Could you check a few things on this drawing? It's one solid part, dimensions in mm from its lowest x, y, z. Give positions to 0.01 mm unless a question says otherwise; leave off trailing zeros. Loops run counter-clockwise (first coordinate to the right, second up) from the corner with the lowest first, then second, coordinate; pieces in that order, holes last.
1. For P1, Ø6, axis at x = 20, z = 6, coming from the -Y side; P2, Ø4, axis at x = 11.5, y = 2.5, coming from the +Z side, each with a flat end and sliding along its axis, tell me the tip position at first contact or that it passes through.
2. Imagine slicing it at D-D (z = 2). List the corners of the cut face in (x, y) for me.
3. Imagine slicing it at C-C (x = 10). List the corners of the cut face in (y, z) for me.
4. I need wall thicknesses on line 1 along Z through (x, y) = (28, 6.5); line 2 along X through (y, z) = (4.5, 1.5); line 3 along Y through (x, z) = (7.5, 13.25). Which ranges of each line are inside material? Lowest first, please.
5. Imagine slicing it at B-B (z = 14.5). List the corners of the cut face in (x, y) for me.
6. Imagine slicing it at A-A (y = 7.25). List the corners of the cut face in (x, z) for me, plus the area to 3 significant figures.
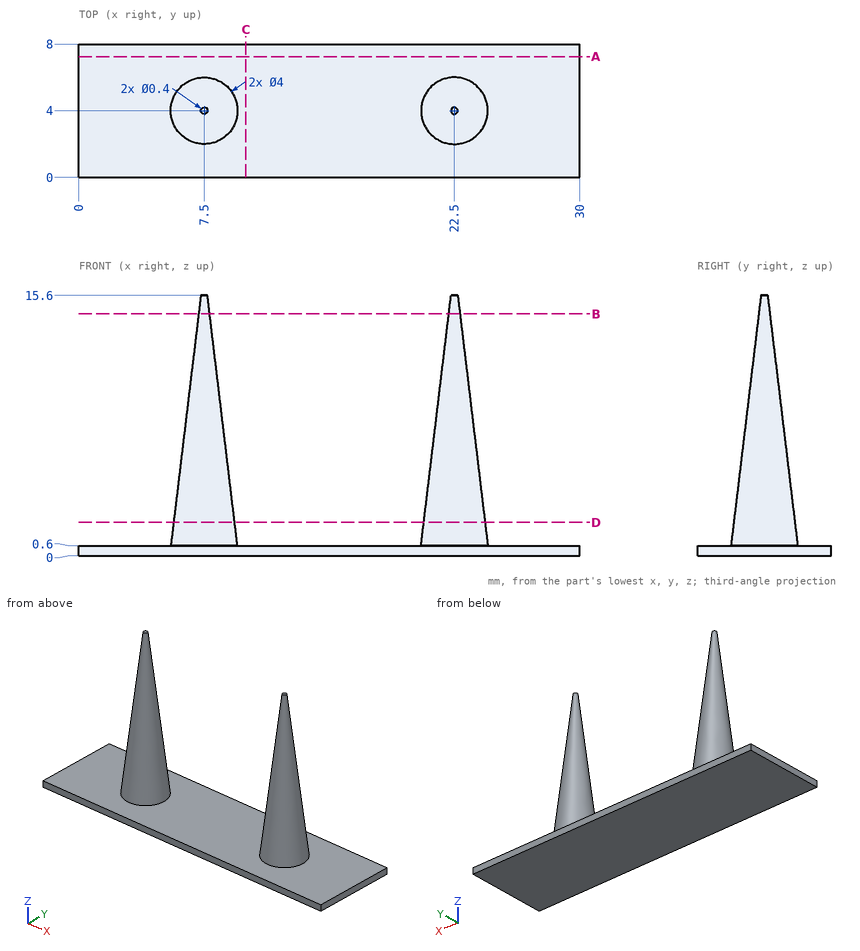
Derived:
1. P1: stops at y = 2.43
1. P2: stops at z = 0.6
2. outline: circle Ø3.66 at (7.5, 4); circle Ø3.66 at (22.5, 4)
3. outline: (0, 0) - (8, 0) - (8, 0.6) - (0, 0.6) - close
4. line 1: z = 0 to 0.6
4. line 2: x = 5.68 to 9.32, 20.68 to 24.32
4. line 3: y = 3.52 to 4.48
5. outline: circle Ø0.66 at (7.5, 4); circle Ø0.66 at (22.5, 4)
6. outline: (0, 0) - (30, 0) - (30, 0.6) - (0, 0.6) - close
6. area: 18.0 mm2
